Autodesk Inventor part; units mm, degrees
ref_plane "YZ Plane" through (0, 0, 0) normal (1, 0, 0) x (0, 1, 0)
ref_plane "XZ Plane" through (0, 0, 0) normal (0, 1, 0) x (-1, 0, 0)
ref_plane "XY Plane" through (0, 0, 0) normal (0, 0, 1) x (1, 0, 0)
sketch "スケッチ1" plane through (0, 0, 0) normal (0, 0, 1) x (1, 0, 0)
  circle A0 centre (0, 0) radius 6
  dimension "d0" = 12
extrude "押し出し1" add sketch "スケッチ1" against normal blind 70
sketch "スケッチ2" plane through (0, 0, 0) normal (0, 0, 1) x (1, 0, 0)
  circle A0 centre (0, 0) radius 6
  circle A1 centre (0, 0) radius 4
  dimension "d3" = 8
extrude "押し出し2" cut sketch "スケッチ2" against normal blind 12.5
sketch "スケッチ3" plane through (0, 0, -70) normal (0, 0, -1) x (-1, 0, 0)
  circle A0 centre (0, 0) radius 6
extrude "押し出し3" add sketch "スケッチ3" along normal blind 3
properties part number "円柱12mm"
Work out the finished part from the listing and answer in its coordinate system (mm). A direction names the side the tool comes from. Coordinates: 2 decimals unless noted, no trailing zeros. Order: outer loops, then holes, each group sorted by start corner. A loop starts at its lowest first (then second) coordinate and runs counter-clockwise, first axis right, second up. Notation, with made-up numbers: (65.25, 20.5) - (77.25, 20.5) arc R15 cw to (77.25, 43.5) - close; hole circle Ø8 at (-5, 58.25). An arc over 180 degrees is marked (long way). Put each result on its own line as item: value. Start each with the question number.
1) Flat-ended cylindrical pins translate along their axes: pin 1 (3 mm diameter, centred on y = 1, z = -10.5, fed in from +X); pin 2 (4 mm diameter, centred on y = 3, z = -36.5, fed in from +X); pin 3 (1.5 mm diameter, centred on y = -2.5, z = -23.5, fed in from +X). Find the tip coordinate at first contact, or state that the pin passes through.
2) Find section C-C (z = -35.5). Give the vertices of the cut face in (x, y), plus the area to 3 significant figures.
3) For faces 1 (the flat face through (-1.42, -3.92, -12.5)), 2 (the cylindrical face through (0, 6, -42)), determine the directions among +Z, -Z, +X, -X, +Y, -Y from which every point of the face is accessible in a straight line to the end or side of a thin tool.
4) Find the intervals of material crossed by line 1 (Z direction, x = 4.5, y = -2.5); line 2 (X direction, y = 2.75, z = -38); line 3 (X direction, y = -0.25, z = -69.5), in increasing order. Write a range as from..to.
5) Find section A-A (x = 0). Give the vertices of the cut face in (y, z), plus the area to 3 significant figures.
6) Find section D-D (y = -5). Give the vertices of the cut face in (x, z), plus the area to 3 significant figures.
Results list:
1. pin 1: stops at x = 4
1. pin 2: stops at x = 5.92
1. pin 3: stops at x = 5.74
2. outline: circle Ø12 at (0, 0)
2. area: 113 mm^2
3. face 1: +Z
3. face 2: +Z, -Z
4. line 1: z = -73..-12.5
4. line 2: x = -5.33..5.33
4. line 3: x = -5.99..5.99
5. outline: (-6, -73) - (6, -73) - (6, -12.5) - (4, -12.5) - (4, 0) - (-4, 0) - (-4, -12.5) - (-6, -12.5) - close
5. area: 826 mm^2
6. outline: (-3.32, -73) - (3.32, -73) - (3.32, -12.5) - (-3.32, -12.5) - close
6. area: 401 mm^2
